Check sheet for the modelled part. Datum: model origin and axes. Units: mm. Face numbers are marked on the shaded views. A direction names the side the tool comes from. Give positions to 0.01 mm unless a question says otherwise; leave off trailing zeros. Write each loop counter-clockwise with the first axis right and the second up, starting at its lowest first coordinate (ties: lowest second). Pieces come first, ordered by that corner, then holes. Notation, with made-up numbers: M 3,77 L 13,77 A21 cw 13,93 Z; hole C 84.25,56.25 d4. An arc over 180 degrees is marked long. Use CSV: the item, a comma, the result in double quotes. Start each with the question number.
1. Depth check by flat-ended pin: P1, Ø6, axis at x = 171.5, z = 207, coming from the +Y side; P2, Ø6, axis at y = -14.5, z = 176.5, coming from the -X side; P3, Ø7.5, axis at y = -9.5, z = 232.5, coming from the +X side; P4, Ø10, axis at x = 270.5, y = -11, coming from the +Z side. Enter the tip coordinate at first touch or a pass-through.
2. Access from +Z, -Z, +X, -X, +Y, -Y to the whole of each face (thin tool, end or side, straight path). Record for the marked faces 1, 2, 3, 4 and 5.
3. Cross-section at A-A, the plane y = -18. Enter the section's corners in (x, z), and give its area (3 significant figures).
4. Cross-section at B-B, the plane z = 229.5. Enter the section's corners in (x, y).
5. Scan lines: line 1 (X direction, y = -4, z = 222); line 2 (X direction, y = -22, z = 180.5). Record each from-to range of solid material in increasing order.
6. Cross-section at C-C, the plane z = 157. Enter the section's corners in (x, y), and give its area (3 significant figures).
from build123d import *

# Parameters (mm, degrees)
F0_W     = 20
F0_H     = 35
F1_DEPTH = 25.4


with BuildPart() as f1:
    # F0 (on Front) → F1 (new body)
    with BuildSketch(Plane.XZ):
        Polygon((-72.583798, 108.904224), (-72.583798, 98.904224), (-52.583798, 98.904224), (-52.583798, 113.904224), align=None)
        Polygon((-52.583798, 113.904224), (-52.583798, 98.904224), (257.416202, 98.904224), (257.416202, 133.904224), (257.416202, 173.904224), (257.416202, 208.904224), (257.416202, 248.904224), (-52.583798, 248.904224), (-52.583798, 233.297413), (-52.583798, 218.297413), (-52.583798, 188.904224), (-52.583798, 168.904224), (-52.583798, 137.904224), align=None)
        with Locations((267.416202, 116.404224)):
            Rectangle(F0_W, F0_H)
        Polygon((-72.583798, 141.323209), (-52.583798, 137.904224), (-52.583798, 168.904224), (-72.583798, 163.323209), align=None)
        with Locations((267.416202, 191.404224)):
            Rectangle(F0_W, F0_H)
        Polygon((-72.583798, 193.904224), (-52.583798, 188.904224), (-52.583798, 218.297413), (-72.583798, 213.904224), align=None)
        Polygon((-52.583798, 233.297413), (-52.583798, 248.904224), (-72.583798, 248.904224), (-72.583798, 238.904224), align=None)
    extrude(amount=F1_DEPTH)


solid = f1.part
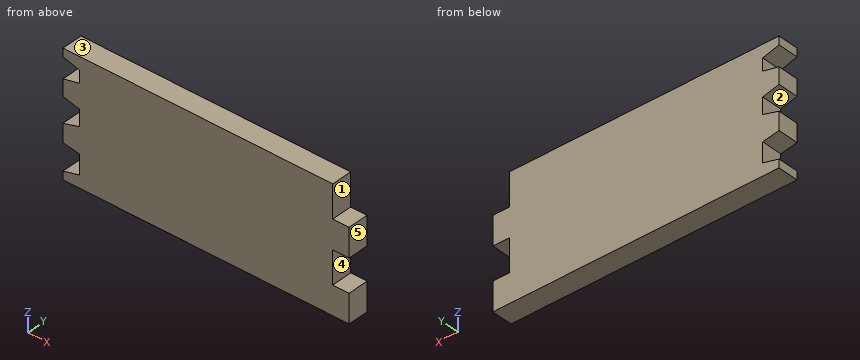
Worked answers:
1,P1,"stops at y = 0"
1,P2,"stops at x = -52.58"
1,P3,"stops at x = 257.42"
1,P4,"stops at z = 208.9"
2,face 1,"+Z, +X, +Y, -Y"
2,face 2,"-X, +Y, -Y"
2,face 3,"+Z, +X, -X, +Y, -Y"
2,face 4,"+X, +Y, -Y"
2,face 5,"+Z, -Z, +X, +Y, -Y"
3,outline,"M -72.58,98.9 L 277.42,98.9 L 277.42,133.9 L 257.42,133.9 L 257.42,173.9 L 277.42,173.9 L 277.42,208.9 L 257.42,208.9 L 257.42,248.9 L -72.58,248.9 L -72.58,238.9 L -52.58,233.3 L -52.58,218.3 L -72.58,213.9 L -72.58,193.9 L -52.58,188.9 L -52.58,168.9 L -72.58,163.32 L -72.58,141.32 L -52.58,137.9 L -52.58,113.9 L -72.58,108.9 Z"
3,area,"49,400 mm^2"
4,outline,"M -52.58,-25.4 L 257.42,-25.4 L 257.42,0 L -52.58,0 Z"
5,line 1,"x = -52.58 to 257.42"
5,line 2,"x = -52.58 to 277.42"
6,outline,"M -72.58,-25.4 L 257.42,-25.4 L 257.42,0 L -72.58,0 Z"
6,area,"8,380 mm^2"
